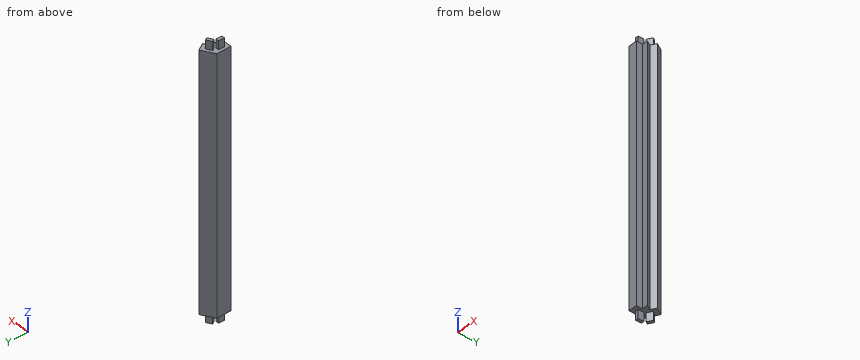
```python
from build123d import *

# Parameters (mm, degrees)
BOSS_EXTRUDE1_DEPTH = 88
SKETCH3_W           = 2
SKETCH3_H           = 2.11
CUT_EXTRUDE1_DEPTH  = 88
CUT_EXTRUDE3_START  = -88
CUT_EXTRUDE3_DEPTH  = 88
SKETCH5_W           = 1
SKETCH5_H           = 2
BOSS_EXTRUDE2_DEPTH = 3
SKETCH6_W           = 1
SKETCH6_H           = 2
BOSS_EXTRUDE3_DEPTH = 3


# Read off the part's stored shape, not the designer's step: Cut-Extrude3
with BuildPart() as part:
    # Sketch1 → Boss-Extrude1 (new body)
    with BuildSketch(Plane.XY):
        Polygon((0, -15.964312624), (-5, -15.964312624), (-5, -10.964312624), (-0.670674615, -8.462924667), (1.830713193, -12.792250104), (0, -13.854312624), align=None)
    extrude(amount=BOSS_EXTRUDE1_DEPTH)

    # Sketch3 → Cut-Extrude1 (cut)
    with BuildSketch(Plane.XY.offset(88)):
        with Locations((-1, -14.909312624)):
            Rectangle(SKETCH3_W, SKETCH3_H)
    extrude(amount=-CUT_EXTRUDE1_DEPTH, mode=Mode.SUBTRACT)

    # Cut-Extrude3 outline → Cut-Extrude3 (cut)
    with BuildSketch(Plane.XY.offset(88).offset(CUT_EXTRUDE3_START)):
        Polygon((0.830158064, -11.060519919), (-1, -12.117944485), (0, -13.854312624), (1.830713193, -12.792250104), align=None)
    extrude(amount=CUT_EXTRUDE3_DEPTH, mode=Mode.SUBTRACT)

    # Sketch5 → Boss-Extrude2 (add)
    with BuildSketch(Plane.XY.offset(88)):
        Polygon((-3.200924793, -11.079761314), (-1.469194639, -10.079206131), (-0.968917048, -10.945071208), (-2.700647202, -11.945626391), align=None)
        with Locations((-3.5, -13.464312624)):
            Rectangle(SKETCH5_W, SKETCH5_H)
    extrude(amount=BOSS_EXTRUDE2_DEPTH)

    # Sketch6 → Boss-Extrude3 (add)
    with BuildSketch(Plane(origin=(0, 0, 0), x_dir=(-1, 0, 0), z_dir=(0, 0, -1))):
        Polygon((1.469194639, -10.079206131), (0.968917048, -10.945071208), (2.700647202, -11.945626391), (3.202395372, -11.080610981), align=None)
        with Locations((3.501951466, -13.465994689)):
            Rectangle(SKETCH6_W, SKETCH6_H)
    extrude(amount=BOSS_EXTRUDE3_DEPTH)


solid = part.part
```
For this review, take the finished solid that the model builds, in its own axes (mm). Give positions to 0.01 mm unless a question says otherwise; leave off trailing zeros. Write each loop counter-clockwise with the first axis right and the second up, starting at its lowest first coordinate (ties: lowest second). Pieces come first, ordered by that corner, then holes.
Item 1: Insertion check: P1, Ø2.5, axis at y = -15, z = 39.5, coming from the +X side; P2, Ø1.6, axis at y = -13.5, z = 89.5, coming from the -X side; P3, Ø2, axis at y = -13.5, z = 90, coming from the +X side; P4, Ø1.5, axis at x = -0.5, z = 41.5, coming from the +Y side. Each pin has a flat end and moves straight along its axis. Give the tip position at first contact, or say it passes through.
Item 2: Wall thickness on probe 1 along X at (y, z) = (-14.25, 46); probe 2 along Z at (x, y) = (-2.4, -10.5); probe 3 along Y at (x, z) = (-0.65, 34): over which ranges is each line inside the solid? List them lowest first.
Item 3: Take a section at A-A (z = 62). Give the boundary of the cut face in (x, y), and give its area (3 significant figures).
Established:
1. P1: stops at x = 0
1. P2: stops at x = -4
1. P3: stops at x = -3
1. P4: stops at y = -8.46
2. probe 1: x = -5 to -2
2. probe 2: z = 0 to 88
2. probe 3: y = -13.85 to -12.73, -11.92 to -8.5
3. outline: (-5, -15.96) - (-2, -15.96) - (-2, -13.85) - (0, -13.85) - (-1, -12.12) - (0.83, -11.06) - (-0.67, -8.46) - (-5, -10.96) - close
3. area: 27.1 mm2
